Check sheet for the modelled part. Datum: model origin and axes. Units: mm. A direction names the side the tool comes from. Round coordinates to 2 decimals unless told otherwise and drop trailing zeros. Order: outer loops, then holes, each group sorted by start corner. A loop starts at its lowest first (then second) coordinate and runs counter-clockwise, first axis right, second up.
Q1. Mould release check, pull along Y, two halves, no side actions. Record for faces 4 (the flat face through (-11, 6, 1.524)), 5 (the cylindrical face through (20.23, 6.37, 9.31)): +Y half, -Y half, draft (parallel to the pull), parting line (faces both ways), or undercut.
Q2. Cross-section at A-A on z = 12.5. Record the cut outline in (x, y), then the cut area to 3 significant figures.
Q3. Set-up check for faces 1 (the flat face through (-0.521, 3, 12)), 2 (the flat face through (0, -2, 17.272)), 3 (the cylindrical face through (-9.549, 9.517, 4.404)): record each of +Z, -Z, +X, -X, +Y, -Y from which the full face is reachable in a straight line by a thin tool's end or side.
Q4. Depth check by flat-ended pin: P1, Ø2.5, axis at x = 1, y = 0.5, coming from the +Z side; P2, Ø0.5, axis at x = -1, z = 13, coming from the -Y side; P3, Ø3, axis at x = 6, y = -11, coming from the -Z side; P4, Ø1.1, axis at x = 12, y = 3, coming from the -Z side. Enter the tip coordinate at first touch or a pass-through.
Q5. Cross-section at C-C on z = 1. Record the cut outline in (x, y), then the cut area to 3 significant figures.
Q6. Scan lines: probe 1 along Y at (x, z) = (0, 6.5); probe 2 along X at (y, z) = (-10, 4); probe 3 along Y at (x, z) = (-5.5, 17.5). Record each from-to range of solid material in increasing order.
from build123d import *

# Parameters (mm, degrees)
SKETCH1_R           = 21.209
SKETCH1_R_2         = 13.208
BOSS_EXTRUDE1_DEPTH = 18.796
FILLET1_R           = 3.175
BOSS_EXTRUDE2_START = -1.524
SKETCH2_R           = 13.208
BOSS_EXTRUDE2_DEPTH = 15.748
SKETCH4_R           = 10.668
SKETCH4_R_2         = 3.937
CUT_EXTRUDE2_DEPTH  = 3.556
CUT_EXTRUDE2_DRAFT  = -10
SKETCH5_R           = 10.668
CUT_EXTRUDE3_DEPTH  = 9.652
SKETCH6_R           = 4.1275
BOSS_EXTRUDE3_DEPTH = 3.81
BOSS_EXTRUDE3_TAPER = 10
CUT_EXTRUDE1_DEPTH  = 20.32
CHAMFER2_SIZE       = 0.683442603
CHAMFER2_SIZE_2     = 2.54
CHAMFER3_SIZE       = 0.683442603
CHAMFER3_SIZE_2     = 2.54
CUT_EXTRUDE4_DEPTH  = 5.842


with BuildPart() as part:
    # Sketch1 → Boss-Extrude1 (new body)
    with BuildSketch(Plane.XY):
        Circle(SKETCH1_R)
        Circle(SKETCH1_R_2, mode=Mode.SUBTRACT)
    extrude(amount=BOSS_EXTRUDE1_DEPTH)

    # Fillet1
    fillet1_edges = [part.edges().sort_by_distance(p)[0] for p in [
        (-21.209, 0, 0),
        (-21.209, 0, 18.796),
    ]]
    fillet(fillet1_edges, radius=FILLET1_R)



with BuildPart() as body_2:
    # Sketch2 → Boss-Extrude2 (new body)
    with BuildSketch(Plane.XY.offset(18.796).offset(BOSS_EXTRUDE2_START)):
        Circle(SKETCH2_R)
    extrude(amount=-BOSS_EXTRUDE2_DEPTH)


with BuildPart() as cut_extrude2_tool:
    # Sketch4 → Cut-Extrude2 (with draft: the straight prism first)
    with BuildSketch(Plane.XY.offset(17.272)):
        Circle(SKETCH4_R)
        Circle(SKETCH4_R_2, mode=Mode.SUBTRACT)
    extrude(amount=-CUT_EXTRUDE2_DEPTH)
    # Cut-Extrude2: the draft: its side faces are tilted about the plane it starts from
    cut_extrude2_sides = [cut_extrude2_tool.faces().sort_by_distance(p)[0] for p in [
        (-10.668, 0, 15.494),
        (-3.937, 0, 15.494),
    ]]
    draft(cut_extrude2_sides, Plane.XY.offset(17.272), CUT_EXTRUDE2_DRAFT)


with BuildPart() as body_2_1:
    add(body_2.part)

    # Cut-Extrude2: cut by cut_extrude2_tool
    add(cut_extrude2_tool.part, mode=Mode.SUBTRACT)

    # Sketch5 → Cut-Extrude3 (cut)
    with BuildSketch(Plane(origin=(0, 0, 1.524), x_dir=(-1, 0, 0), z_dir=(0, 0, -1))):
        Circle(SKETCH5_R)
    extrude(amount=-CUT_EXTRUDE3_DEPTH, mode=Mode.SUBTRACT)


with BuildPart() as part_1:
    add(part.part)

    add(body_2_1.part)  # Boss-Extrude3 merges body 2
    # Sketch6 → Boss-Extrude3 (add)
    with BuildSketch(Plane(origin=(0, 0, 11.176), x_dir=(-1, 0, 0), z_dir=(0, 0, -1))):
        Circle(SKETCH6_R)
    extrude(amount=BOSS_EXTRUDE3_DEPTH, taper=BOSS_EXTRUDE3_TAPER)

    # Sketch3 → Cut-Extrude1 (cut)
    with BuildSketch(Plane.XY.offset(17.272)):
        with BuildLine():
            Line((-1.17021598, 0.9384), (-0.5207, 0.9384))
            Line((-0.5207, 0.9384), (-0.5207, 6.710804028))
            Line((-0.5207, 6.710804028), (0.5207, 6.710804028))
            Line((0.5207, 6.710804028), (0.5207, 0.9384))
            Line((0.5207, 0.9384), (1.17021598, 0.9384))
            ThreePointArc((1.17021598, 0.9384), (0, -1.5), (-1.17021598, 0.9384))
        make_face()
    extrude(amount=-CUT_EXTRUDE1_DEPTH, mode=Mode.SUBTRACT)

    # Chamfer2
    # the kernel refuses this chamfer: 2.54, 0.683442603 mm, written as the material it takes off along each edge
    with BuildSketch(Plane(origin=(0, 0, 18.796), x_dir=(1, 0, 0), z_dir=(0, -1, 0))) as chamfer2_piece_1_section:
        Polygon((13.208 + CHAMFER2_SIZE, 0), (13.208, -CHAMFER2_SIZE_2), (13.208, 0), align=None)
    chamfer2_piece_1 = revolve(axis=Axis((0, 0, 18.796), (0, 0, 1)), mode=Mode.PRIVATE)
    chamfer2_piece_1 = split(chamfer2_piece_1, bisect_by=Plane(origin=(-13.659448533, 0, 17.272), z_dir=(0, 0, 1)), keep=Keep.TOP, mode=Mode.PRIVATE)
    add(chamfer2_piece_1, mode=Mode.SUBTRACT)

    # Chamfer3
    # the kernel refuses this chamfer: 2.54, 0.683442603 mm, written as the material it takes off along each edge
    with BuildSketch(Plane(origin=(0, 0, 0), x_dir=(1, 0, 0), z_dir=(0, -1, 0))) as chamfer3_piece_1_section:
        Polygon((13.208 + CHAMFER3_SIZE, 0), (13.208, CHAMFER3_SIZE_2), (13.208, 0), align=None)
    chamfer3_piece_1 = revolve(axis=Axis((0, 0, 0), (0, 0, 1)), mode=Mode.PRIVATE)
    chamfer3_piece_1 = split(chamfer3_piece_1, bisect_by=Plane(origin=(-13.659448521, 0, 1.524), z_dir=(0, 0, -1)), keep=Keep.TOP, mode=Mode.PRIVATE)
    add(chamfer3_piece_1, mode=Mode.SUBTRACT)

    # Sketch8 → Cut-Extrude4 (cut)
    with BuildSketch(Plane(origin=(0, 0, 1.524), x_dir=(-1, 0, 0), z_dir=(0, 0, -1))):
        with BuildLine():
            Line((1.931554123, 13.34228712), (0.26745284, 7.131776584))
            Line((0.26745284, 7.131776584), (3.334267338, 6.310026116))
            Line((3.334267338, 6.310026116), (4.998368621, 12.520536652))
            ThreePointArc((4.998368621, 12.520536652), (3.489237132, 13.022010258), (1.931554123, 13.34228712))
        make_face()
        with BuildLine():
            Line((8.343918499, 10.588982529), (3.797509246, 6.042573276))
            Line((3.797509246, 6.042573276), (6.042573276, 3.797509246))
            Line((6.042573276, 3.797509246), (10.588982529, 8.343918499))
            ThreePointArc((10.588982529, 8.343918499), (9.532773125, 9.532773125), (8.343918499, 10.588982529))
        make_face()
        with BuildLine():
            Line((12.520536652, 4.998368621), (6.310026116, 3.334267338))
            Line((6.310026116, 3.334267338), (7.131776584, 0.26745284))
            Line((7.131776584, 0.26745284), (13.34228712, 1.931554123))
            ThreePointArc((13.34228712, 1.931554123), (13.022010258, 3.489237132), (12.520536652, 4.998368621))
        make_face()
        with BuildLine():
            Line((13.34228712, -1.931554123), (7.131776584, -0.26745284))
            Line((7.131776584, -0.26745284), (6.310026116, -3.334267338))
            Line((6.310026116, -3.334267338), (12.520536652, -4.998368621))
            ThreePointArc((12.520536652, -4.998368621), (13.022010258, -3.489237132), (13.34228712, -1.931554123))
        make_face()
        with BuildLine():
            Line((10.588982529, -8.343918499), (6.042573276, -3.797509246))
            Line((6.042573276, -3.797509246), (3.797509246, -6.042573276))
            Line((3.797509246, -6.042573276), (8.343918499, -10.588982529))
            ThreePointArc((8.343918499, -10.588982529), (9.532773125, -9.532773125), (10.588982529, -8.343918499))
        make_face()
        with BuildLine():
            Line((4.998368621, -12.520536652), (3.334267338, -6.310026116))
            Line((3.334267338, -6.310026116), (0.26745284, -7.131776584))
            Line((0.26745284, -7.131776584), (1.931554123, -13.34228712))
            ThreePointArc((1.931554123, -13.34228712), (3.489237132, -13.022010258), (4.998368621, -12.520536652))
        make_face()
        with BuildLine():
            Line((-1.931554123, -13.34228712), (-0.26745284, -7.131776584))
            Line((-0.26745284, -7.131776584), (-3.334267338, -6.310026116))
            Line((-3.334267338, -6.310026116), (-4.998368621, -12.520536652))
            ThreePointArc((-4.998368621, -12.520536652), (-3.489237132, -13.022010258), (-1.931554123, -13.34228712))
        make_face()
        with BuildLine():
            Line((-8.343918499, -10.588982529), (-3.797509246, -6.042573276))
            Line((-3.797509246, -6.042573276), (-6.042573276, -3.797509246))
            Line((-6.042573276, -3.797509246), (-10.588982529, -8.343918499))
            ThreePointArc((-10.588982529, -8.343918499), (-9.532773125, -9.532773125), (-8.343918499, -10.588982529))
        make_face()
        with BuildLine():
            Line((-12.520536652, -4.998368621), (-6.310026116, -3.334267338))
            Line((-6.310026116, -3.334267338), (-7.131776584, -0.26745284))
            Line((-7.131776584, -0.26745284), (-13.34228712, -1.931554123))
            ThreePointArc((-13.34228712, -1.931554123), (-13.022010258, -3.489237132), (-12.520536652, -4.998368621))
        make_face()
        with BuildLine():
            Line((-13.34228712, 1.931554123), (-7.131776584, 0.26745284))
            Line((-7.131776584, 0.26745284), (-6.310026116, 3.334267338))
            Line((-6.310026116, 3.334267338), (-12.520536652, 4.998368621))
            ThreePointArc((-12.520536652, 4.998368621), (-13.022010258, 3.489237132), (-13.34228712, 1.931554123))
        make_face()
        with BuildLine():
            Line((-10.588982529, 8.343918499), (-6.042573276, 3.797509246))
            Line((-6.042573276, 3.797509246), (-3.797509246, 6.042573276))
            Line((-3.797509246, 6.042573276), (-8.343918499, 10.588982529))
            ThreePointArc((-8.343918499, 10.588982529), (-9.532773125, 9.532773125), (-10.588982529, 8.343918499))
        make_face()
        with BuildLine():
            Line((-4.998368621, 12.520536652), (-3.334267338, 6.310026116))
            Line((-3.334267338, 6.310026116), (-0.26745284, 7.131776584))
            Line((-0.26745284, 7.131776584), (-1.931554123, 13.34228712))
            ThreePointArc((-1.931554123, 13.34228712), (-3.489237132, 13.022010258), (-4.998368621, 12.520536652))
        make_face()
    extrude(amount=-CUT_EXTRUDE4_DEPTH, mode=Mode.SUBTRACT)


solid = part_1.part
Results found:
1. face 4: undercut
1. face 5: parting line
2. outline: circle Ø42.42 at (0, 0); hole (-1.17, 0.94) arc R1.5 ccw (long way) to (1.17, 0.94) - (0.52, 0.94) - (0.52, 6.71) - (-0.52, 6.71) - (-0.52, 0.94) - close
2. area: 1,400 mm2
3. face 1: +Z, -Z
3. face 2: +Z
3. face 3: -Z
4. P1: stops at z = 17.27
4. P2: stops at y = -21.2
4. P3: stops at z = 0
4. P4: stops at z = 7.37
5. outline: circle Ø40.69 at (0, 0); hole circle Ø27.24 at (0, 0)
5. area: 718 mm2
6. probe 1: y = -21.21 to -10.67, 10.67 to 21.21
6. probe 2: x = -18.7 to -9.04, -7.75 to -4.32, 4.32 to 7.75, 9.04 to 18.7
6. probe 3: y = -19.85 to -12.38, 12.38 to 19.85
